from build123d import *

# Parameters (mm, degrees)
SKETCH_1_R          = 25
SKETCH_1_R_2        = 2
EXTRUDE_1_DEPTH     = 2
EXTRUDE_START       = -2
EXTRUDE_2_DEPTH     = 2
SKETCH_3_R          = 13.5
CUT_EXTRUDE_1_DEPTH = 2


with BuildPart() as part:
    # 草图1 → 凸台-拉伸1 (new body)
    with BuildSketch(Plane.XY):
        Circle(SKETCH_1_R)
        with Locations((0, 17.5)):
            Circle(SKETCH_1_R_2, mode=Mode.SUBTRACT)
        with Locations((17.5, 0)):
            Circle(SKETCH_1_R_2, mode=Mode.SUBTRACT)
        with Locations((0, -17.5)):
            Circle(SKETCH_1_R_2, mode=Mode.SUBTRACT)
        with Locations((-17.5, 0)):
            Circle(SKETCH_1_R_2, mode=Mode.SUBTRACT)
    extrude(amount=EXTRUDE_1_DEPTH)

    # 草图2 → 凸台-拉伸2 (add)
    with BuildSketch(Plane.XY.offset(2).offset(EXTRUDE_START)):
        with BuildLine():
            Line((-10, 22.912878475), (-10, 37.912878475))
            Line((-10, 37.912878475), (-3.05, 37.912878475))
            Line((-3.05, 37.912878475), (-3.05, 30))
            ThreePointArc((-3.05, 30), (0, 26.95), (3.05, 30))
            Line((3.05, 30), (3.05, 37.912878475))
            Line((3.05, 37.912878475), (10, 37.912878475))
            Line((10, 37.912878475), (10, 22.912878475))
            ThreePointArc((10, 22.912878475), (0, 25), (-10, 22.912878475))
        make_face()
    extrude(amount=EXTRUDE_2_DEPTH)

    # 草图3 → 切除-拉伸1 (cut)
    with BuildSketch(Plane.XY.offset(2)):
        Circle(SKETCH_3_R)
    extrude(amount=-CUT_EXTRUDE_1_DEPTH, mode=Mode.SUBTRACT)


solid = part.part
Geometry check sheet. Reference: the model listing, model coordinates, mm. A direction names the side the tool comes from. Give positions to 0.01 mm unless a question says otherwise; leave off trailing zeros. Write each loop counter-clockwise with the first axis right and the second up, starting at its lowest first coordinate (ties: lowest second). Pieces come first, ordered by that corner, then holes.
1) Cross-section at C-C (x = 9). Record the boundary of the cut face in (y, z).
Values follow:
outline: (-23.32, 0) - (-10.06, 0) - (-10.06, 2) - (-23.32, 2) - close; (10.06, 0) - (37.91, 0) - (37.91, 2) - (10.06, 2) - close
2) Cross-section at B-B (y = 4.5). Record the boundary of the cut face in (x, z), plus the area to 3 significant figures.
Values follow:
outline: (-24.59, 0) - (-12.73, 0) - (-12.73, 2) - (-24.59, 2) - close; (12.73, 0) - (24.59, 0) - (24.59, 2) - (12.73, 2) - close
area: 47.5 mm2
3) Go/stop test with flat-tipped pins: pin 1 Ø0.6 at (y, z) = (35, 1) entering from -X; pin 2 Ø0.6 at (y, z) = (34.5, 0.5) entering from +X. Record where each tip stops, or that it passes through.
Values follow:
pin 1: stops at x = -10
pin 2: stops at x = 10
4) Set-up check for faces 4 (the face through (3.05, 34, 1)), 5 (the face through (15.9, -1.2, 1)), 6 (the face through (10, 31, 1)): record each of +Z, -Z, +X, -X, +Y, -Y from which the full face is reachable in a straight line by a thin tool's end or side.
Values follow:
face 4: +Z, -Z, +Y
face 5: +Z, -Z
face 6: +Z, -Z, +X, +Y
5) Cross-section at A-A (z = 0.45). Record the boundary of the cut face in (x, y), plus the area to 3 significant figures.
Values follow:
outline: (-10, 22.91) arc R25 ccw (long way) to (10, 22.91) - (10, 37.91) - (3.05, 37.91) - (3.05, 30) arc R3.05 cw to (-3.05, 30) - (-3.05, 37.91) - (-10, 37.91) - close; hole circle Ø4 at (-17.5, 0); hole circle Ø27 at (0, 0); hole circle Ø4 at (0, -17.5); hole circle Ø4 at (0, 17.5); hole circle Ø4 at (17.5, 0)
area: 1,550 mm2
6) Thickness scan on line 1 (Y direction, x = 0, z = 1.3); line 2 (X direction, y = 33.5, z = 1.85); line 3 (X direction, y = -6.5, z = 0.2). Record the ranges inside material, lowest first.
Values follow:
line 1: y = -25 to -19.5, -15.5 to -13.5, 13.5 to 15.5, 19.5 to 26.95
line 2: x = -10 to -3.05, 3.05 to 10
line 3: x = -24.14 to -11.83, 11.83 to 24.14
7) Release check for a two-part mould opening along Y. For faces 1 (the face through (-2.93, -13.18, 1.01)), 2 (the face through (-10, 30, 1)), 3 (the face through (-0.07, 26.95, 0.99)) record: released by +Y, released by -Y, zero draft, split by the parting line, or undercut.
Values follow:
face 1: undercut
face 2: zero draft
face 3: released by +Y
